The model under review builds one solid part; all positions refer to its coordinate system, in mm. Face numbers are marked on the shaded views. A direction names the side the tool comes from. Round coordinates to 2 decimals unless told otherwise and drop trailing zeros. Loops run counter-clockwise (first coordinate to the right, second up) from the corner with the lowest first, then second, coordinate; pieces in that order, holes last. Notation, with made-up numbers: (21, 60.25) -> (25, 60.25) arc R26 cw to (25, 99.25) -> close; hole circle Ø7 at (56.25, 14.25). An arc over 180 degrees is marked (long way). Write each question's results on one line, items separated by ' | '. Start each with the question number.
Item 1: Clearance check with flat-ended pins moving along their axes: pin 1 Ø3 at (x, y) = (-5, 18) entering from +Z; pin 2 Ø10 at (x, z) = (-1.5, -9) entering from +Y; pin 3 Ø6.5 at (x, y) = (4.5, 11) entering from +Z; pin 4 Ø1.5 at (x, z) = (0.5, -2) entering from +Y. State where each tip first meets the part, or that it passes through.
Item 2: For L1, parallel to X at y = 2.5, z = -10; L2, parallel to Z at x = -8.25, y = 21; L3, parallel to X at y = 11.5, z = 0, list the stretches that pass through material, from the lowest coordinate up. Write a range as from..to.
Item 3: Mouldability with a two-part tool opening along X and no side actions: class the marked faces 1, 2 and 3 as pulls with the +X half, pulls with the -X half, needs draft (parallel to the pull), parting line crosses it, or undercut.
Item 4: Tool access review of the marked faces 4, 5 and 6: name each direction out of +Z, -Z, +X, -X, +Y, -Y from which nothing blocks a thin tool from reaching the whole face with its end or side.
Item 5: We need section C-C (z = -31). Give the boundary of the cut face in (x, y), and give its area (3 significant figures).
Item 6: We need section A-A (z = 5.5). Give the boundary of the cut face in (x, y).
Item 7: We need section B-B (z = -8). Give the boundary of the cut face in (x, y), and give its area (3 significant figures).
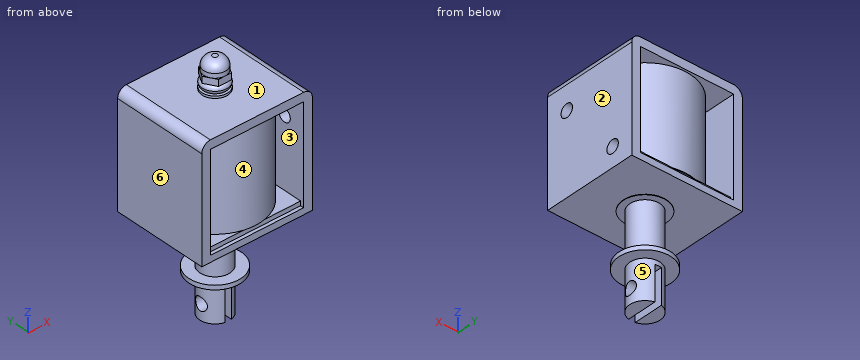
from build123d import *

# Parameters (mm, degrees)
SKETCH2_W               = 25.5
SKETCH2_H               = 26
BOSS_EXTRUDE1_DEPTH     = 22
FILLET1_R               = 2
SKETCH3_W               = 21.5
SKETCH3_H               = 22.5
CUT_EXTRUDE1_DEPTH      = 22
SKETCH4_W               = 21.5
SKETCH4_H               = 20.4
BOSS_EXTRUDE2_DEPTH     = 1
SKETCH5_R               = 10.5
BOSS_EXTRUDE3_DEPTH     = 21.5
SKETCH7_R               = 3
BOSS_EXTRUDE4_DEPTH     = 0.5
SKETCH8_R               = 3
BOSS_EXTRUDE5_DEPTH     = 2
SKETCH7_3_R             = 3
CUT_EXTRUDE2_DEPTH      = 0.5
FILLET2_R               = 1
FILLET3_R               = 1
SKETCH7_4_R             = 3
BOSS_EXTRUDE6_DEPTH     = 0.5
BOSS_EXTRUDE7_DEPTH     = 1.5
SKETCH10_R              = 2.6
BOSS_EXTRUDE8_DEPTH     = 3
FILLET4_R               = 2
SKETCH11_R              = 3.5
BOSS_EXTRUDE9_DEPTH     = 11.5
SKETCH12_R              = 6
BOSS_EXTRUDE10_DEPTH    = 1
SKETCH13_R              = 3.5
BOSS_EXTRUDE11_DEPTH    = 9
SKETCH15_W              = 1.5
SKETCH15_H              = 7
CUT_EXTRUDE3_DEPTH      = 8
CUT_EXTRUDE4_DEPTH      = 5
CUT_EXTRUDE4_DEPTH_BACK = 5
SKETCH16_R              = 1.5
SKETCH17_R              = 5
CUT_EXTRUDE5_DEPTH      = 2
SKETCH18_R              = 5
BOSS_EXTRUDE14_DEPTH    = 2.1
SKETCH19_R              = 1.5
CUT_EXTRUDE6_DEPTH      = 2


with BuildPart() as part:
    # Sketch2 → Boss-Extrude1 (new body)
    with BuildSketch(Plane(origin=(0, 0, 0), x_dir=(1, 0, 0), z_dir=(0, 1, 0))):
        Rectangle(SKETCH2_W, SKETCH2_H)
    extrude(amount=BOSS_EXTRUDE1_DEPTH)

    # Fillet1
    fillet1_edges = [part.edges().sort_by_distance(p)[0] for p in [
        (12.75, 11, 13),
        (-12.75, 11, 13),
    ]]
    fillet(fillet1_edges, radius=FILLET1_R)

    # Sketch3 → Cut-Extrude1 (cut)
    with BuildSketch(Plane(origin=(0, 22, 0), x_dir=(1, 0, 0), z_dir=(0, 1, 0))):
        with Locations((0, 0.25)):
            Rectangle(SKETCH3_W, SKETCH3_H)
    extrude(amount=-CUT_EXTRUDE1_DEPTH, mode=Mode.SUBTRACT)

    # Sketch4 → Boss-Extrude2 (add)
    with BuildSketch(Plane.XY.offset(-11.5)):
        with Locations((0, 11)):
            Rectangle(SKETCH4_W, SKETCH4_H)
    extrude(amount=BOSS_EXTRUDE2_DEPTH)

    # Sketch5 → Boss-Extrude3 (add)
    with BuildSketch(Plane.XY.offset(-10.5)):
        with Locations(Location((0, 11, 0), (0, 0, 256.270867325))):
            Circle(SKETCH5_R)
    extrude(amount=BOSS_EXTRUDE3_DEPTH)

    # Sketch7 → Boss-Extrude4 (add)
    with BuildSketch(Plane.XY.offset(13)):
        with Locations(Location((0, 11, 0), (0, 0, 180))):
            Circle(SKETCH7_R)
    extrude(amount=BOSS_EXTRUDE4_DEPTH)

    # Sketch8 → Boss-Extrude5 (add)
    with BuildSketch(Plane.XY.offset(13.5)):
        with Locations(Location((0, 11, 0), (0, 0, 180))):
            Circle(SKETCH8_R)
    extrude(amount=BOSS_EXTRUDE5_DEPTH)

    # Sketch7<3> → Cut-Extrude2 (cut)
    with BuildSketch(Plane.XY.offset(13)):
        with Locations((0, 11)):
            Circle(SKETCH7_3_R)
    extrude(amount=CUT_EXTRUDE2_DEPTH, mode=Mode.SUBTRACT)


with BuildPart() as cut_extrude2_piece_1:
    # of the separate pieces the step leaves, piece 1, a body of its own (cut_extrude2_pieces)
    add(part.part.solids().sort_by_distance((-10.75, 0, 13))[0])



with BuildPart() as cut_extrude2_piece_2:
    # of the separate pieces the step leaves, piece 2, a body of its own (cut_extrude2_pieces)
    add(part.part.solids().sort_by_distance((-3, 11, 13.5))[0])

    # Fillet2
    fillet2_edges = [cut_extrude2_piece_2.edges().sort_by_distance(p)[0] for p in [
        (3, 11, 13.5),
    ]]
    fillet(fillet2_edges, radius=FILLET2_R)

    # Fillet3
    fillet3_edges = [cut_extrude2_piece_2.edges().sort_by_distance(p)[0] for p in [
        (3, 11, 15.5),
    ]]
    fillet(fillet3_edges, radius=FILLET3_R - 0.0001)  # a hair under: the kernel refuses the full size


with BuildPart() as cut_extrude2_piece_1_1:
    add(cut_extrude2_piece_1.part)

    add(cut_extrude2_piece_2.part)  # Boss-Extrude6 merges Cut-Extrude2 piece 2
    # Sketch7<4> → Boss-Extrude6 (add)
    with BuildSketch(Plane.XY.offset(13)):
        with Locations(Location((0, 11, 0), (0, 0, 180))):
            Circle(SKETCH7_4_R)
    extrude(amount=BOSS_EXTRUDE6_DEPTH)

    # Sketch9 → Boss-Extrude7 (add)
    with BuildSketch(Plane.XY.offset(15.5)):
        Polygon((3.0022214, 11), (1.5011107, 13.6), (-1.5011107, 13.6), (-3.0022214, 11), (-1.5011107, 8.4), (1.5011107, 8.4), align=None)
    extrude(amount=BOSS_EXTRUDE7_DEPTH)

    # Sketch10 → Boss-Extrude8 (add)
    with BuildSketch(Plane.XY.offset(17)):
        with Locations(Location((0, 11, 0), (0, 0, 150))):
            Circle(SKETCH10_R)
    extrude(amount=BOSS_EXTRUDE8_DEPTH)

    # Fillet4
    fillet4_edges = [cut_extrude2_piece_1_1.edges().sort_by_distance(p)[0] for p in [
        (2.25166605, 9.7, 20),
    ]]
    fillet(fillet4_edges, radius=FILLET4_R)

    # Sketch11 → Boss-Extrude9 (add)
    with BuildSketch(Plane(origin=(0, 0, -13), x_dir=(-1, 0, 0), z_dir=(0, 0, -1))):
        with Locations((0, 11)):
            Circle(SKETCH11_R)
    extrude(amount=BOSS_EXTRUDE9_DEPTH)

    # Sketch12 → Boss-Extrude10 (add)
    with BuildSketch(Plane(origin=(0, 0, -24.5), x_dir=(-1, 0, 0), z_dir=(0, 0, -1))):
        with Locations((0, 11)):
            Circle(SKETCH12_R)
    extrude(amount=BOSS_EXTRUDE10_DEPTH)

    # Sketch13 → Boss-Extrude11 (add)
    with BuildSketch(Plane(origin=(0, 0, -25.5), x_dir=(-1, 0, 0), z_dir=(0, 0, -1))):
        with Locations((0, 11)):
            Circle(SKETCH13_R)
    extrude(amount=BOSS_EXTRUDE11_DEPTH)

    # Sketch15 → Cut-Extrude3 (cut)
    with BuildSketch(Plane(origin=(0, 0, -34.5), x_dir=(-1, 0, 0), z_dir=(0, 0, -1))):
        with Locations((0, 11)):
            Rectangle(SKETCH15_W, SKETCH15_H)
    extrude(amount=-CUT_EXTRUDE3_DEPTH, mode=Mode.SUBTRACT)

    # Sketch16 → Cut-Extrude4 (cut, two sides: drawn at the far end of the back side and taken through both)
    with BuildSketch(Plane.ZY.offset(-0.75).offset(-CUT_EXTRUDE4_DEPTH_BACK)):
        with Locations(Location((-31, 10.922268779, 0), (0, 0, 180))):
            Circle(SKETCH16_R)
    extrude(amount=CUT_EXTRUDE4_DEPTH + CUT_EXTRUDE4_DEPTH_BACK, mode=Mode.SUBTRACT)

    # Sketch17 → Cut-Extrude5 (cut)
    with BuildSketch(Plane(origin=(0, 0, -13), x_dir=(-1, 0, 0), z_dir=(0, 0, -1))):
        with Locations((0, 11)):
            Circle(SKETCH17_R)
    extrude(amount=-CUT_EXTRUDE5_DEPTH, mode=Mode.SUBTRACT)


with BuildPart() as cut_extrude5_piece_1:
    # of the separate pieces the step leaves, piece 1, a body of its own (cut_extrude5_pieces)
    add(cut_extrude2_piece_1_1.part.solids().sort_by_distance((12.75, 0, -13))[0])



with BuildPart() as cut_extrude5_piece_2:
    # of the separate pieces the step leaves, piece 2, a body of its own (cut_extrude5_pieces)
    add(cut_extrude2_piece_1_1.part.solids().sort_by_distance((-6, 11, -24.5))[0])


with BuildPart() as cut_extrude5_piece_1_1:
    add(cut_extrude5_piece_1.part)

    add(cut_extrude5_piece_2.part)  # Boss-Extrude14 merges Cut-Extrude5 piece 2
    # Sketch18 → Boss-Extrude14 (add)
    with BuildSketch(Plane(origin=(0, 0, -11), x_dir=(-1, 0, 0), z_dir=(0, 0, -1))):
        with Locations((0, 11)):
            Circle(SKETCH18_R)
    extrude(amount=BOSS_EXTRUDE14_DEPTH)

    # Sketch19 → Cut-Extrude6 (cut)
    with BuildSketch(Plane(origin=(12.75, 0, 0), x_dir=(0, 0, -1), z_dir=(1, 0, 0))):
        with Locations((-5.5, 5)):
            Circle(SKETCH19_R)
        with Locations((8.5, 17)):
            Circle(SKETCH19_R)
    extrude(amount=-CUT_EXTRUDE6_DEPTH, mode=Mode.SUBTRACT)


solid = cut_extrude5_piece_1_1.part
Here are the results:
1) pin 1: stops at z = 13 | pin 2: stops at y = 22 | pin 3: stops at z = 19.89 | pin 4: stops at y = 21.5
2) L1: x = -12.75..-10.75, -6.16..6.16, 10.75..12.75 | L2: z = -13..-10.5, 11..13 | L3: x = -12.75..-10.75, -10.49..10.49, 10.75..12.75
3) face 1: needs draft | face 2: pulls with the +X half | face 3: undercut
4) face 4: none | face 5: -Z | face 6: +Z, -Z, -X, +Y, -Y
5) outline: (-3.2, 12.42) -> (-0.75, 12.42) -> (-0.75, 14.42) arc R3.5 ccw to start; (-3.12, 9.42) arc R3.5 ccw to (-0.75, 7.58) -> (-0.75, 9.42) -> close; (0.75, 7.58) arc R3.5 ccw to (3.12, 9.42) -> (0.75, 9.42) -> close; (0.75, 12.42) -> (3.2, 12.42) arc R3.5 ccw to (0.75, 14.42) -> close | area: 12.2 mm2
6) outline: (-12.75, 0) -> (-10.75, 0) -> (-10.75, 22) -> (-12.75, 22) -> close; circle Ø21 at (0, 11); (10.75, 0) -> (12.75, 0) -> (12.75, 3.5) -> (10.75, 3.5) -> close; (10.75, 6.5) -> (12.75, 6.5) -> (12.75, 22) -> (10.75, 22) -> close
7) outline: (-12.75, 0) -> (-10.75, 0) -> (-10.75, 22) -> (-12.75, 22) -> close; circle Ø21 at (0, 11); (10.75, 0) -> (12.75, 0) -> (12.75, 15.59) -> (10.75, 15.59) -> close; (10.75, 18.41) -> (12.75, 18.41) -> (12.75, 22) -> (10.75, 22) -> close | area: 429 mm2
